from build123d import *

# Parameters (mm, degrees)
SKETCH1_W             = 40
SKETCH1_H             = 50
BOSS_EXTRUDE1_DEPTH   = 4
SKETCH2_W             = 24
SKETCH2_H             = 58
BOSS_EXTRUDE2_DEPTH   = 8
SKETCH4_W             = 24
SKETCH4_H             = 58
BOSS_EXTRUDE3_DEPTH   = 8
BOSS_EXTRUDE5_DEPTH   = 40
SKETCH6_W             = 32
SKETCH6_H             = 50
CUT_EXTRUDE1_DEPTH    = 8
M5_TAPPED_HOLE3_D     = 4.2
M5_TAPPED_HOLE3_DEPTH = 8
M5_TAPPED_HOLE4_D     = 4.2
M5_TAPPED_HOLE5_D     = 4.2
M5_TAPPED_HOLE5_DEPTH = 8


with BuildPart() as part:
    # Sketch1 → Boss-Extrude1 (new, symmetric)
    with BuildSketch(Plane.XY):
        Rectangle(SKETCH1_W, SKETCH1_H)
    extrude(amount=BOSS_EXTRUDE1_DEPTH, both=True)

    # Sketch2 → Boss-Extrude2 (add)
    with BuildSketch(Plane(origin=(20, 0, 0), x_dir=(0, 0, -1), z_dir=(1, 0, 0))):
        with Locations((8, 4)):
            Rectangle(SKETCH2_W, SKETCH2_H)
    extrude(amount=BOSS_EXTRUDE2_DEPTH)

    # Sketch4 → Boss-Extrude3 (add)
    with BuildSketch(Plane.ZY.offset(20)):
        with Locations((-8, 4)):
            Rectangle(SKETCH4_W, SKETCH4_H)
    extrude(amount=BOSS_EXTRUDE3_DEPTH)

    # Sketch5 → Boss-Extrude5 (add)
    with BuildSketch(Plane.ZY.offset(-20)):
        Polygon((-20, -25), (-20, 33), (4, 33), (4, 25), (-12.05, 25), (-12.05, -25), align=None)
    extrude(amount=BOSS_EXTRUDE5_DEPTH)

    # Sketch6 → Cut-Extrude1 (cut)
    with BuildSketch(Plane(origin=(0, 0, -20), x_dir=(-1, 0, 0), z_dir=(0, 0, -1))):
        Rectangle(SKETCH6_W, SKETCH6_H)
    extrude(amount=-CUT_EXTRUDE1_DEPTH, mode=Mode.SUBTRACT)

    # M5 Tapped Hole3
    with Locations(Plane(origin=(0, 0, -4), x_dir=(-1, 0, 0), z_dir=(0, 0, -1))):
        with Locations((-17, 22), (17, 22), (17, -3), (-17, -3)):
            Hole(M5_TAPPED_HOLE3_D / 2, depth=M5_TAPPED_HOLE3_DEPTH)

    # M5 Tapped Hole4 (through all)
    with Locations(Plane(origin=(0, 33, 0), x_dir=(1, 0, 0), z_dir=(0, 1, 0))):
        with Locations((0, 8)):
            Hole(M5_TAPPED_HOLE4_D / 2)

    # M5 Tapped Hole5
    with Locations(Plane(origin=(28, 0, 0), x_dir=(0, 0, -1), z_dir=(1, 0, 0))):
        with Locations((8.025, 15), (8.025, 0), (8.025, -15)):
            Hole(M5_TAPPED_HOLE5_D / 2, depth=M5_TAPPED_HOLE5_DEPTH)


solid = part.part
The listing builds one solid part. Answer for the finished solid, in the listing's coordinates (mm). A direction names the side the tool comes from. Coordinates: 2 decimals unless noted, no trailing zeros. Write each loop counter-clockwise with the first axis right and the second up, starting at its lowest first coordinate (ties: lowest second). Pieces come first, ordered by that corner, then holes. Notation, with made-up numbers: (9, 53) - (39, 53) arc R14 cw to (39, 71) - close; hole circle Ø7 at (53.5, -14.5). An arc over 180 degrees is marked (long way). Answer as CSV lines item,"result".
1. Find section D-D (y = 22). Give the vertices of the cut face in (x, z).
Computed values:
outline,"(-28, -20) - (-16, -20) - (-16, -12.05) - (-20, -12.05) - (-20, -4) - (-19.1, -4) - (-19.1, 4) - (-28, 4) - close; (-14.9, -4) - (14.9, -4) - (14.9, 4) - (-14.9, 4) - close; (16, -20) - (28, -20) - (28, 4) - (19.1, 4) - (19.1, -4) - (20, -4) - (20, -12.05) - (16, -12.05) - close"
2. A tool of negligible diameter and unlimited length cuts with its end or side. For faces 1 (the flat face through (-20, 0, -8)), 2 (the cylindrical face through (-14.997, -2.369, 0.056)), 3 (the cylindrical face through (23.944, 16.771, -6.896)), from which of +Z, -Z, +X, -X, +Y, -Y can it reach the whole face along a straight path? Write none if from no direction.
Computed values:
face 1,"-Y"
face 2,"+Z"
face 3,"+X"
3. Find section B-B (x = 17). Give the vertices of the cut face in (y, z), plus the area to 3 significant figures.
Computed values:
outline,"(-25, -20) - (33, -20) - (33, 4) - (24.1, 4) - (24.1, -4) - (25, -4) - (25, -12.05) - (-25, -12.05) - close; (-25, -4) - (-5.1, -4) - (-5.1, 4) - (-25, 4) - close; (-0.9, -4) - (19.9, -4) - (19.9, 4) - (-0.9, 4) - close"
area,"922 mm²"
4. Find section C-C (z = -7.25). Give the vertices of the cut face in (x, y).
Computed values:
outline,"(-28, -25) - (-20, -25) - (-20, 25) - (-1.96, 25) - (-1.96, 33) - (-28, 33) - close; (1.96, 25) - (20, 25) - (20, 16.95) - (28, 16.95) - (28, 33) - (1.96, 33) - close; (20, -25) - (28, -25) - (28, -16.95) - (20, -16.95) - close; (20, -13.05) - (28, -13.05) - (28, -1.95) - (20, -1.95) - close; (20, 1.95) - (28, 1.95) - (28, 13.05) - (20, 13.05) - close"
5. Find section A-A (y = -15). Give the vertices of the cut face in (x, z) (3 decimals), plus the area to 3 significant figures.
Computed values:
outline,"(-28, -20) - (-16, -20) - (-16, -12.05) - (-20, -12.05) - (-20, -4) - (20, -4) - (20, -5.925) - (28, -5.925) - (28, 4) - (-28, 4) - close; (16, -20) - (28, -20) - (28, -10.125) - (20, -10.125) - (20, -12.05) - (16, -12.05) - close"
area,"734 mm²"
6. Straight lines are drawn through the part: line 1 (Y direction, x = 17, z = 0.25); line 2 (Z direction, x = 0, y = 29.5); line 3 (X direction, y = 6.5, z = -15.75). For each, find the intervals that lie inside material, in ascending order. Write a range as [from, to].
Computed values:
line 1,"y = [-25, -5.1], [-0.9, 19.9], [24.1, 33]"
line 2,"z = [-20, -10.1], [-5.9, 4]"
line 3,"x = [-28, -16], [16, 28]"
7. Given P1, Ø3.5, axis at y = 15, z = -8.025, coming from the +X side; P2, Ø6, axis at x = -4, z = -14, coming from the -Y side; P3, Ø12, axis at x = -12.5, y = 24, coming from the -Z side; P4, Ø20, axis at x = -5, y = 4, coming from the -Z side, each flat-ended and moving along its own axis, determine where each tip first touches the part or whether it passes through.
Computed values:
P1,"stops at x = -20"
P2,"stops at y = 25"
P3,"stops at z = -20"
P4,"stops at z = -4"
8. Determine the mould class of faces 4 (the flat face through (16, 0, -16)), 5 (the flat face through (-28, 4, -8)), 6 (the flat face through (0, -25, -2)) for opening direction X: +X half, -X half, draft (parallel to the pull), parting line (faces both ways), or undercut.
Computed values:
face 4,"undercut"
face 5,"-X half"
face 6,"draft"
